For this review, take the finished solid that the model builds, in its own axes (mm). Face numbers are marked on the shaded views. A direction names the side the tool comes from. Give positions to 0.01 mm unless a question says otherwise; leave off trailing zeros. Write each loop counter-clockwise with the first axis right and the second up, starting at its lowest first coordinate (ties: lowest second). Pieces come first, ordered by that corner, then holes.
1) We need section B-B on x = -72. Give the boundary of the cut face in (y, z), and give its area (3 significant figures).
2) We need section A-A on z = -55.5. Give the boundary of the cut face in (x, y).
3) We need section D-D on z = -35.5. Give the boundary of the cut face in (x, y).
4) Machinability: for the marked faces 1, 2, 3 and 4, which of the approach directions +Z, -Z, +X, -X, +Y, -Y give a long, thin tool a straight path to every point of the face, cutting with its end or side? Answer none if there is none.
5) Draft analysis for pull direction Z (two halves, no side actions). For the marked faces 5, 6, 7 and 8, state which applies: pulls with the +Z half, pulls with the -Z half, needs draft (parallel to the pull), parting line crosses it, or undercut.
6) We need section C-C on y = 35.5. Give the boundary of the cut face in (x, z).
7) Wall thickness on line 1 along X through (y, z) = (-3.5, -9); line 2 along Z through (x, y) = (-64, 26); line 3 along X through (y, z) = (69.5, -6): over which ranges is each line inside the solid? List them lowest first.
8) For P1, Ø4, axis at x = -70, y = 41.5, coming from the +Z side; P2, Ø6.5, axis at x = -8, z = 3.5, coming from the +Y side; P3, Ø13, axis at x = -67.5, y = -5, coming from the -Z side, all flat-tipped, find the tip position at first contact; note any pin that passes through.
from build123d import *

# Parameters (mm, degrees)
BOSS_EXTRUDE3_DEPTH  = 125
SKETCH3_W            = 125
SKETCH3_H            = 69.296464556
BOSS_EXTRUDE5_DEPTH  = 12
CUT_EXTRUDE1_DEPTH   = 159.836393815
SKETCH7_W            = 105
SKETCH7_H            = 10
BOSS_EXTRUDE6_DEPTH  = 8
SKETCH8_W            = 105
SKETCH8_H            = 10
BOSS_EXTRUDE7_DEPTH  = 8
SKETCH9_W            = 105
SKETCH9_H            = 55.154328932
CUT_EXTRUDE2_DEPTH   = 161.78246173
SKETCH11_W           = 10
SKETCH11_H           = 55.154328932
CUT_EXTRUDE3_DEPTH   = 6
SKETCH12_W           = 10
SKETCH12_H           = 55.154328932
CUT_EXTRUDE4_DEPTH   = 6
SKETCH13_W           = 105
SKETCH13_H           = 61.154328932
CUT_EXTRUDE6_DEPTH   = 3
SKETCH14_R           = 1.9
CUT_EXTRUDE8_DEPTH   = 6
SKETCH15_R           = 1.9
CUT_EXTRUDE9_DEPTH   = 6
BOSS_EXTRUDE9_REACH  = 158.4
SKETCH25_W           = 10
SKETCH25_H           = 6
BOSS_EXTRUDE13_DEPTH = 10
CUT_EXTRUDE10_DEPTH  = 1
CUT_EXTRUDE11_DEPTH  = 1
SKETCH29_W           = 11
SKETCH29_H           = 81.296464556
BOSS_EXTRUDE15_DEPTH = 6
SKETCH31_R           = 2
CUT_EXTRUDE16_DEPTH  = 6
SKETCH32_R           = 2
CUT_EXTRUDE17_DEPTH  = 6
CUT_EXTRUDE22_DEPTH  = 157.400127877
CUT_EXTRUDE23_DEPTH  = 157.400127877


with BuildPart() as part:
    # Sketch1 → Boss-Extrude3 (new body)
    with BuildSketch(Plane(origin=(0, 0, 0), x_dir=(0, 0, -1), z_dir=(1, 0, 0))):
        Polygon((0, 0), (69.296464556, 0), (0, 69.296464556), align=None)
    extrude(amount=-BOSS_EXTRUDE3_DEPTH)

    # Sketch3 → Boss-Extrude5 (add)
    with BuildSketch(Plane.XZ):
        with Locations((-62.5, -34.648232278)):
            Rectangle(SKETCH3_W, SKETCH3_H)
    extrude(amount=BOSS_EXTRUDE5_DEPTH)

    # Sketch6 → Cut-Extrude1 (cut, through all)
    with BuildSketch(Plane.ZY.offset(125)):
        Polygon((-7.071067812, 62.225396744), (-62.225396744, 7.071067812), (-7.071067812, 7.071067812), align=None)
    extrude(amount=-CUT_EXTRUDE1_DEPTH, mode=Mode.SUBTRACT)

    # Sketch7 → Boss-Extrude6 (add)
    with BuildSketch(Plane(origin=(0, 34.648232278, -34.648232278), x_dir=(1, 0, 0), z_dir=(0, 0.7071067811865515, -0.7071067811865436))):
        with Locations((-62.5, 44)):
            Rectangle(SKETCH7_W, SKETCH7_H)
    extrude(amount=BOSS_EXTRUDE6_DEPTH)

    # Sketch8 → Boss-Extrude7 (add)
    with BuildSketch(Plane(origin=(0, 34.648232278, -34.648232278), x_dir=(1, 0, 0), z_dir=(0, 0.7071067811865515, -0.7071067811865436))):
        with Locations((-62.5, -44)):
            Rectangle(SKETCH8_W, SKETCH8_H)
    extrude(amount=BOSS_EXTRUDE7_DEPTH)

    # Sketch9 → Cut-Extrude2 (cut, through all)
    with BuildSketch(Plane(origin=(0, 7.071067812, 0), x_dir=(1, 0, 0), z_dir=(0, 1, 0))):
        with Locations((-62.5, 34.648232278)):
            Rectangle(SKETCH9_W, SKETCH9_H)
    extrude(amount=-CUT_EXTRUDE2_DEPTH, mode=Mode.SUBTRACT)

    # Sketch11 → Cut-Extrude3 (cut)
    with BuildSketch(Plane(origin=(0, 7.071067812, 0), x_dir=(1, 0, 0), z_dir=(0, 1, 0))):
        with Locations((-5, 34.648232278)):
            Rectangle(SKETCH11_W, SKETCH11_H)
    extrude(amount=-CUT_EXTRUDE3_DEPTH, mode=Mode.SUBTRACT)

    # Sketch12 → Cut-Extrude4 (cut)
    with BuildSketch(Plane(origin=(0, 7.071067812, 0), x_dir=(1, 0, 0), z_dir=(0, 1, 0))):
        with Locations((-120, 34.648232278)):
            Rectangle(SKETCH12_W, SKETCH12_H)
    extrude(amount=-CUT_EXTRUDE4_DEPTH, mode=Mode.SUBTRACT)

    # Sketch13 → Cut-Extrude6 (cut)
    with BuildSketch(Plane(origin=(0, 0, -7.071067812), x_dir=(-1, 0, 0), z_dir=(0, 0, -1))):
        with Locations((62.5, 31.648232278)):
            Rectangle(SKETCH13_W, SKETCH13_H)
    extrude(amount=-CUT_EXTRUDE6_DEPTH, mode=Mode.SUBTRACT)

    # Sketch14 → Cut-Extrude8 (cut)
    with BuildSketch(Plane(origin=(0, 34.648232278, -34.648232278), x_dir=(1, 0, 0), z_dir=(0, 0.7071067811865515, -0.7071067811865436))):
        with Locations(Location((-6.25, 42.75, 0), (0, 0, 270))):
            Circle(SKETCH14_R)
    cut_extrude8 = extrude(amount=-CUT_EXTRUDE8_DEPTH, mode=Mode.SUBTRACT)

    # Mirror1: Cut-Extrude8 across plane
    add(cut_extrude8.mirror(Plane(origin=(-62.5, 0, 0), x_dir=(0, 0, 1), z_dir=(1, 0, 0))), mode=Mode.SUBTRACT)

    # Sketch15 → Cut-Extrude9 (cut)
    with BuildSketch(Plane(origin=(0, 34.648232278, -34.648232278), x_dir=(1, 0, 0), z_dir=(0, 0.7071067811865515, -0.7071067811865436))):
        with Locations(Location((-6.25, -42.75, 0), (0, 0, 270))):
            Circle(SKETCH15_R)
    cut_extrude9 = extrude(amount=-CUT_EXTRUDE9_DEPTH, mode=Mode.SUBTRACT)

    # Mirror2: Cut-Extrude9 across plane
    add(cut_extrude9.mirror(Plane(origin=(-62.5, 0, 0), x_dir=(0, 0, 1), z_dir=(1, 0, 0))), mode=Mode.SUBTRACT)

    # Sketch22 → Boss-Extrude9 (add, up to next)
    with BuildSketch(Plane.ZY.offset(10), mode=Mode.PRIVATE) as boss_extrude9_sk1:
        Polygon((-7.071067812, 62.225396744), (-4.071067812, 59.225396744), (-4.071067812, 62.225396744), align=None)
    boss_extrude9_tool1 = extrude(boss_extrude9_sk1.sketch, amount=BOSS_EXTRUDE9_REACH, mode=Mode.PRIVATE) - part.part
    add(boss_extrude9_tool1.solids().sort_by_distance((-10, 61.225397, -5.071068))[0])

    # Sketch25 → Boss-Extrude13 (add)
    with BuildSketch(Plane.XY.offset(-62.225396744)):
        with Locations((-5, 4.071067812)):
            Rectangle(SKETCH25_W, SKETCH25_H)
        with Locations((-120, 4.071067812)):
            Rectangle(SKETCH25_W, SKETCH25_H)
    extrude(amount=BOSS_EXTRUDE13_DEPTH)

    # Sketch26 → Cut-Extrude10 (cut)
    with BuildSketch(Plane(origin=(-10, 0, 0), x_dir=(0, 0, -1), z_dir=(1, 0, 0))):
        Polygon((0, 69.296464556), (7.071067812, 62.225396744), (12.727922061, 67.882250994), (5.656854249, 74.953318806), align=None)
    cut_extrude10 = extrude(amount=-CUT_EXTRUDE10_DEPTH, mode=Mode.SUBTRACT)

    # Sketch27 → Cut-Extrude11 (cut)
    with BuildSketch(Plane(origin=(-10, 0, 0), x_dir=(0, 0, -1), z_dir=(1, 0, 0))):
        Polygon((62.225396744, 7.071067812), (69.296464556, 0), (74.953318806, 5.656854249), (67.882250994, 12.727922061), align=None)
    cut_extrude11 = extrude(amount=-CUT_EXTRUDE11_DEPTH, mode=Mode.SUBTRACT)

    # Mirror3: Cut-Extrude10, Cut-Extrude11 across plane
    add(cut_extrude10.mirror(Plane(origin=(-62.5, 0, 0), x_dir=(0, 0, 1), z_dir=(1, 0, 0))), mode=Mode.SUBTRACT)
    add(cut_extrude11.mirror(Plane(origin=(-62.5, 0, 0), x_dir=(0, 0, 1), z_dir=(1, 0, 0))), mode=Mode.SUBTRACT)

    # Sketch29 → Boss-Extrude15 (add)
    with BuildSketch(Plane.XY):
        with Locations((-5.5, 28.648232278)):
            Rectangle(SKETCH29_W, SKETCH29_H)
    boss_extrude15 = extrude(amount=BOSS_EXTRUDE15_DEPTH)

    # Mirror4: Boss-Extrude15 across plane
    add(boss_extrude15.mirror(Plane(origin=(-62.5, 0, 0), x_dir=(0, 0, 1), z_dir=(1, 0, 0))))

    # Sketch31 → Cut-Extrude16 (cut)
    with BuildSketch(Plane(origin=(0, 34.648232278, -34.648232278), x_dir=(1, 0, 0), z_dir=(0, 0.7071067811865513, -0.7071067811865438))):
        with Locations(Location((-6.25, 42.75, 0), (0, 0, 270))):
            Circle(SKETCH31_R)
    cut_extrude16 = extrude(amount=-CUT_EXTRUDE16_DEPTH, mode=Mode.SUBTRACT)

    # Sketch32 → Cut-Extrude17 (cut)
    with BuildSketch(Plane(origin=(0, 34.648232278, -34.648232278), x_dir=(1, 0, 0), z_dir=(0, 0.7071067811865513, -0.7071067811865438))):
        with Locations(Location((-6.25, -42.75, 0), (0, 0, 270))):
            Circle(SKETCH32_R)
    cut_extrude17 = extrude(amount=-CUT_EXTRUDE17_DEPTH, mode=Mode.SUBTRACT)

    # Mirror5: Cut-Extrude16, Cut-Extrude17 across plane
    add(cut_extrude16.mirror(Plane(origin=(-62.5, 0, 0), x_dir=(0, 0, 1), z_dir=(1, 0, 0))), mode=Mode.SUBTRACT)
    add(cut_extrude17.mirror(Plane(origin=(-62.5, 0, 0), x_dir=(0, 0, 1), z_dir=(1, 0, 0))), mode=Mode.SUBTRACT)

    # Sketch41 → Cut-Extrude22 (cut, through all)
    with BuildSketch(Plane.ZY.offset(10)):
        Polygon((-7.071067812, 1.071067812), (-4.071067812, 1.071067812), (-4.071067812, 59.225396744), (-7.071067812, 62.225396744), align=None)
    extrude(amount=-CUT_EXTRUDE22_DEPTH, mode=Mode.SUBTRACT)

    # Sketch42 → Cut-Extrude23 (cut, through all)
    with BuildSketch(Plane(origin=(-115, 0, 0), x_dir=(0, 0, -1), z_dir=(1, 0, 0))):
        Polygon((7.071067812, 1.071067812), (4.071067812, 1.071067812), (4.071067812, 59.225396744), (7.071067812, 62.225396744), align=None)
    extrude(amount=-CUT_EXTRUDE23_DEPTH, mode=Mode.SUBTRACT)


solid = part.part
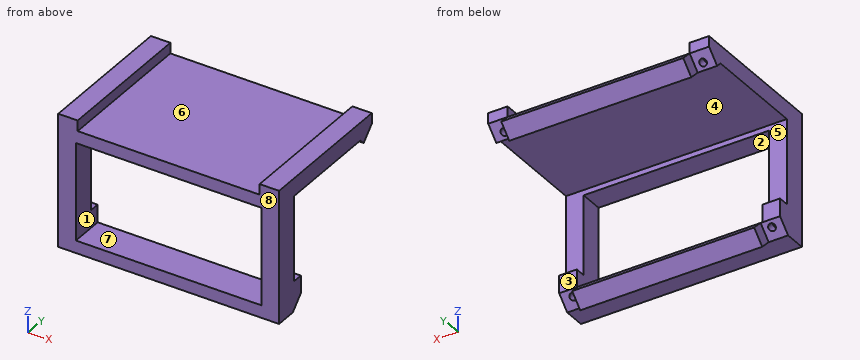
Results list:
1. outline: (-12, -69.3) - (0, -69.3) - (5.66, -74.95) - (12.73, -67.88) - (7.07, -62.23) - (-12, -62.23) - close; (-12, -7.07) - (1.07, -7.07) - (1.07, -4.07) - (59.23, -4.07) - (67.88, -12.73) - (74.95, -5.66) - (69.3, 0) - (-12, 0) - close
1. area: 641 mm2
2. outline: (-125, -12) - (-115, -12) - (-115, 7.07) - (-125, 7.07) - close; (-10, -12) - (0, -12) - (0, 7.07) - (-10, 7.07) - close
3. outline: (-125, -12) - (-115, -12) - (-115, 1.07) - (-125, 1.07) - close; (-10, -12) - (0, -12) - (0, 1.07) - (-10, 1.07) - close
4. face 1: +Y, -Y
4. face 2: -Y
4. face 3: -Z, +X, -X, +Y
4. face 4: +X, -X
5. face 5: undercut
5. face 6: pulls with the +Z half
5. face 7: undercut
5. face 8: needs draft
6. outline: (-125, -4.07) - (0, -4.07) - (0, 6) - (-11, 6) - (-11, 0) - (-114, 0) - (-114, 6) - (-125, 6) - close
7. line 1: x = -125 to -115, -10 to 0
7. line 2: z = -4.07 to 0
7. line 3: x = -114 to -11
8. P1: stops at z = 0
8. P2: stops at y = 69.3
8. P3: stops at z = -70.8
